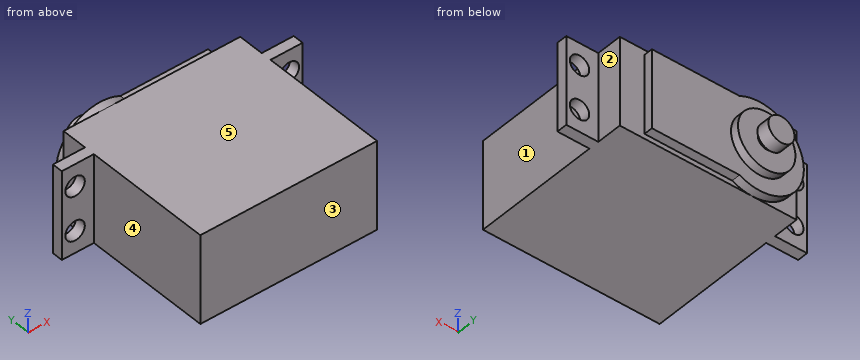
from build123d import *

# Parameters (mm, degrees)
SKETCH_1_W      = 40
SKETCH_1_H      = 20
EXTRUDE_1_DEPTH = 37
EXTRUDE_START   = -5.8
SKETCH_2_W      = 54.5
SKETCH_2_H      = 20
SKETCH_2_R      = 2.2
EXTRUDE_2_DEPTH = 2.4
EXTRUDE_3_DEPTH = 2
SKETCH_4_R      = 6.5
EXTRUDE_4_DEPTH = 1.9
SKETCH_5_R      = 2
EXTRUDE_5_DEPTH = 4
SKETCH_6_R      = 2.95
EXTRUDE_6_DEPTH = 3


with BuildPart() as part:
    # 草图1 → 凸台-拉伸1 (new body)
    with BuildSketch(Plane(origin=(0, 0, 0), x_dir=(1, 0, 0), z_dir=(0, 1, 0))):
        Rectangle(SKETCH_1_W, SKETCH_1_H)
    extrude(amount=EXTRUDE_1_DEPTH)

    # 草图2 → 凸台-拉伸2 (add)
    with BuildSketch(Plane(origin=(0, 37, 0), x_dir=(1, 0, 0), z_dir=(0, 1, 0)).offset(EXTRUDE_START)):
        Rectangle(SKETCH_2_W, SKETCH_2_H)
        with Locations(Location((24.25, 5, 0), (0, 0, 270))):
            Circle(SKETCH_2_R, mode=Mode.SUBTRACT)
        with Locations(Location((24.25, -5, 0), (0, 0, 270))):
            Circle(SKETCH_2_R, mode=Mode.SUBTRACT)
        with Locations(Location((-24.25, 5, 0), (0, 0, 270))):
            Circle(SKETCH_2_R, mode=Mode.SUBTRACT)
        with Locations(Location((-24.25, -5, 0), (0, 0, 270))):
            Circle(SKETCH_2_R, mode=Mode.SUBTRACT)
    extrude(amount=-EXTRUDE_2_DEPTH)

    # 草图3 → 凸台-拉伸3 (add)
    with BuildSketch(Plane(origin=(0, 37, 0), x_dir=(1, 0, 0), z_dir=(0, 1, 0))):
        with BuildLine():
            Line((-5.440394754, 8.9), (14.4, 8.9))
            Line((14.4, 8.9), (14.4, -8.9))
            Line((14.4, -8.9), (-5.440394754, -8.9))
            ThreePointArc((-5.440394754, -8.9), (-20, 0), (-5.440394754, 8.9))
        make_face()
    extrude(amount=EXTRUDE_3_DEPTH)

    # 草图4 → 凸台-拉伸4 (add)
    with BuildSketch(Plane(origin=(0, 39, 0), x_dir=(1, 0, 0), z_dir=(0, 1, 0))):
        with Locations(Location((-10, 0, 0), (0, 0, 90))):
            Circle(SKETCH_4_R)
    extrude(amount=EXTRUDE_4_DEPTH)

    # 草图5 → 凸台-拉伸5 (add)
    with BuildSketch(Plane(origin=(0, 40.9, 0), x_dir=(1, 0, 0), z_dir=(0, 1, 0))):
        with Locations(Location((-10, 0, 0), (0, 0, 270))):
            Circle(SKETCH_5_R)
    extrude(amount=EXTRUDE_5_DEPTH)

    # 草图6 → 凸台-拉伸6 (add)
    with BuildSketch(Plane(origin=(0, 44.9, 0), x_dir=(1, 0, 0), z_dir=(0, 1, 0))):
        with Locations(Location((-10, 0, 0), (0, 0, 270))):
            Circle(SKETCH_6_R)
    extrude(amount=-EXTRUDE_6_DEPTH)


solid = part.part
Could you check a few things on this model? Use its own coordinates, in mm. Face numbers are marked on the shaded views. A direction names the side the tool comes from. Round coordinates to 2 decimals unless told otherwise and drop trailing zeros. Write each loop counter-clockwise with the first axis right and the second up, starting at its lowest first coordinate (ties: lowest second). Pieces come first, ordered by that corner, then holes. Notation, with made-up numbers: (45.5, -2) - (78.5, -2) arc R24 cw to (78.5, 16) - close; hole circle Ø6 at (28, 49.25). An arc over 180 degrees is marked (long way). Use a Markdown table: item, result.
Q1. I want a section at C-C (x = 12). List the corners of the cut face in (y, z) for me.
Output values:
| item | result |
|---|---|
| outline | (0, -10) - (37, -10) - (37, -8.9) - (39, -8.9) - (39, 8.9) - (37, 8.9) - (37, 10) - (0, 10) - close |
Q2. I want a section at D-D (z = 4.25). List the corners of the cut face in (x, y) for me.
Output values:
| item | result |
|---|---|
| outline | (-27.25, 28.8) - (-26.32, 28.8) - (-26.32, 31.2) - (-27.25, 31.2) - close; (-22.18, 28.8) - (-20, 28.8) - (-20, 0) - (20, 0) - (20, 28.8) - (22.18, 28.8) - (22.18, 31.2) - (20, 31.2) - (20, 37) - (14.4, 37) - (14.4, 39) - (-5.08, 39) - (-5.08, 40.9) - (-14.92, 40.9) - (-14.92, 39) - (-19.05, 39) - (-19.05, 37) - (-20, 37) - (-20, 31.2) - (-22.18, 31.2) - close; (26.32, 28.8) - (27.25, 28.8) - (27.25, 31.2) - (26.32, 31.2) - close |
Q3. Please list where these lines run through material, in increasing order: L1, parallel to Z at x = 24, y = 29; L2, parallel to X at y = 30, z = 5; L3, parallel to X at y = 10.5, z = -8.
Output values:
| item | result |
|---|---|
| L1 | -10 to -7.19, -2.81 to 2.81, 7.19 to 10 |
| L2 | -27.25 to -26.45, -22.05 to 22.05, 26.45 to 27.25 |
| L3 | -20 to 20 |
Q4. I want a section at A-A (x = -24.25). List the corners of the cut face in (y, z) for me.
Output values:
| item | result |
|---|---|
| outline | (28.8, -10) - (31.2, -10) - (31.2, -7.2) - (28.8, -7.2) - close; (28.8, -2.8) - (31.2, -2.8) - (31.2, 2.8) - (28.8, 2.8) - close; (28.8, 7.2) - (31.2, 7.2) - (31.2, 10) - (28.8, 10) - close |
Q5. For pin 1 (3 mm diameter, centred on y = 35.5, z = -3, fed in from +X); pin 2 (3 mm diameter, centred on y = 34, z = 4.5, fed in from -X); pin 3 (3.5 mm diameter, centred on x = -23.5, z = -5, fed in from +Y), each with a flat end and sliding along its axis, tell me the tip position at first contact or that it passes through.
Output values:
| item | result |
|---|---|
| pin 1 | x = 20 |
| pin 2 | x = -20 |
| pin 3 | y = 31.2 |
Q6. For the marked faces 1, 2, 3, 4 and 5, which set-ups out of +Z, -Z, +X, -X, +Y, -Y let a thin tool reach every point of the face, with its end or its side?
Output values:
| item | result |
|---|---|
| face 1 | +Z, -Z, +X, -Y |
| face 2 | +Z, -Z, +X, +Y |
| face 3 | +Z, -Z, +X, -X, -Y |
| face 4 | +Z, -Z, -X, -Y |
| face 5 | +Z, +X, -X, +Y, -Y |
Q7. I want a section at B-B (z = -5). List the corners of the cut face in (x, y) for me.
Output values:
| item | result |
|---|---|
| outline | (-27.25, 28.8) - (-26.45, 28.8) - (-26.45, 31.2) - (-27.25, 31.2) - close; (-22.05, 28.8) - (-20, 28.8) - (-20, 0) - (20, 0) - (20, 28.8) - (22.05, 28.8) - (22.05, 31.2) - (20, 31.2) - (20, 37) - (14.4, 37) - (14.4, 39) - (-5.85, 39) - (-5.85, 40.9) - (-14.15, 40.9) - (-14.15, 39) - (-18.66, 39) - (-18.66, 37) - (-20, 37) - (-20, 31.2) - (-22.05, 31.2) - close; (26.45, 28.8) - (27.25, 28.8) - (27.25, 31.2) - (26.45, 31.2) - close |
